Design review of the part built by this model. Coordinates are the model's own, in mm. Face numbers are marked on the shaded views. A direction names the side the tool comes from. Round coordinates to 2 decimals unless told otherwise and drop trailing zeros. Write each loop counter-clockwise with the first axis right and the second up, starting at its lowest first coordinate (ties: lowest second). Pieces come first, ordered by that corner, then holes.
from build123d import *

# Parameters (mm, degrees)
SCHIZZO1_R                   = 4
ESTRUSIONE_ESTRUSIONE1_DEPTH = 4
SCHIZZO2_R                   = 1.5
TAGLIO_ESTRUSIONE1_DEPTH     = 5
SCHIZZO3_R                   = 3.5
SCHIZZO3_R_2                 = 2
TAGLIO_ESTRUSIONE2_DEPTH     = 0.25
SCHIZZO4_R                   = 3
SCHIZZO4_R_2                 = 2
TAGLIO_ESTRUSIONE3_DEPTH     = 0.1
SCHIZZO5_R                   = 4.75
SCHIZZO5_R_2                 = 4
ESTRUSIONE_ESTRUSIONE2_DEPTH = 1
SCHIZZO6_W                   = 0.2
SCHIZZO6_H                   = 0.8


with BuildPart() as part:
    # Schizzo1 → Estrusione-Estrusione1 (new body)
    with BuildSketch(Plane.XY):
        Circle(SCHIZZO1_R)
    extrude(amount=ESTRUSIONE_ESTRUSIONE1_DEPTH)

    # Schizzo2 → Taglio-Estrusione1 (cut, through all)
    with BuildSketch(Plane.XY.offset(4)):
        Circle(SCHIZZO2_R)
    extrude(amount=-TAGLIO_ESTRUSIONE1_DEPTH, mode=Mode.SUBTRACT)

    # Schizzo3 → Taglio-Estrusione2 (cut)
    with BuildSketch(Plane(origin=(0, 0, 0), x_dir=(-1, 0, 0), z_dir=(0, 0, -1))):
        Circle(SCHIZZO3_R)
        Circle(SCHIZZO3_R_2, mode=Mode.SUBTRACT)
    taglio_estrusione2 = extrude(amount=-TAGLIO_ESTRUSIONE2_DEPTH, mode=Mode.SUBTRACT)

    # Schizzo4 → Taglio-Estrusione3 (cut)
    with BuildSketch(Plane(origin=(0, 0, 0.25), x_dir=(-1, 0, 0), z_dir=(0, 0, -1))):
        Circle(SCHIZZO4_R)
        Circle(SCHIZZO4_R_2, mode=Mode.SUBTRACT)
    taglio_estrusione3 = extrude(amount=-TAGLIO_ESTRUSIONE3_DEPTH, mode=Mode.SUBTRACT)

    # Specchia1: Taglio-Estrusione2, Taglio-Estrusione3 across plane
    add(taglio_estrusione2.mirror(Plane.XY.offset(2)), mode=Mode.SUBTRACT)
    add(taglio_estrusione3.mirror(Plane.XY.offset(2)), mode=Mode.SUBTRACT)

    # Schizzo5 → Estrusione-Estrusione2 (add)
    with BuildSketch(Plane.XY):
        Circle(SCHIZZO5_R)
        Circle(SCHIZZO5_R_2, mode=Mode.SUBTRACT)
    extrude(amount=ESTRUSIONE_ESTRUSIONE2_DEPTH)

    # Schizzo6 → Taglia-Rivoluzione1 (revolve, cut)
    with BuildSketch(Plane(origin=(0, 0, 0), x_dir=(1, 0, 0), z_dir=(0, 1, 0))):
        with Locations((3.9, -1.4)):
            Rectangle(SCHIZZO6_W, SCHIZZO6_H)
    revolve(axis=Axis((0, 0, 4), (0, 0, -1)), mode=Mode.SUBTRACT)


solid = part.part
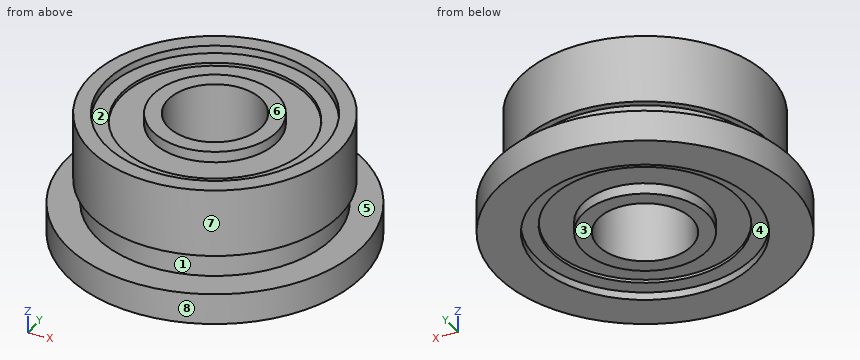
1) The part is to be moulded in two halves that separate along Y. For the marked faces 1, 2 and 3, say which applies: pulls with the +Y half, pulls with the -Y half, needs draft (parallel to the pull), parting line crosses it, or undercut.
2) For the marked faces 4, 5, 6, 7 and 8, list the 3-axis set-ups (+Z, -Z, +X, -X, +Y, -Y) from which the entire face can be reached by the end or side of a thin tool; tool diameter is ignored.
3) Add section B-B on z = 0.6. State the section outline as (x, y) points.
4) Add section C-C on z = 1.4. State the section outline as (x, y) points.
5) For line 1 along Y through (x, z) = (0, 0.3); line 2 along Y through (x, z) = (0, 3.9); line 3 along Y through (x, z) = (0, 2.05), list the stretches that pass through material, from the lowest coordinate up.
6) Add section A-A on y = -2.75. State the section outline as (x, z) points.
7) For P1, Ø1.5, axis at x = -2, z = 2.5, coming from the -Y side, flat-tipped, find the tip position at first contact; note if it passes through.
Computed:
1. face 1: parting line crosses it
1. face 2: undercut
1. face 3: needs draft
2. face 4: -Z
2. face 5: none
2. face 6: +Z, +X, -X, +Y, -Y
2. face 7: +Z
2. face 8: +Z, -Z
3. outline: circle Ø9.5 at (0, 0); hole circle Ø3 at (0, 0)
4. outline: circle Ø7.6 at (0, 0); hole circle Ø3 at (0, 0)
5. line 1: y = -4.75 to -3, -2 to -1.5, 1.5 to 2, 3 to 4.75
5. line 2: y = -4 to -3.5, -2 to -1.5, 1.5 to 2, 3.5 to 4
5. line 3: y = -4 to -1.5, 1.5 to 4
6. outline: (-3.87, 0) - (-2.17, 0) - (-2.17, 0.25) - (-1.2, 0.25) - (-1.2, 0.35) - (1.2, 0.35) - (1.2, 0.25) - (2.17, 0.25) - (2.17, 0) - (3.87, 0) - (3.87, 1) - (2.62, 1) - (2.62, 1.8) - (2.9, 1.8) - (2.9, 4) - (2.17, 4) - (2.17, 3.75) - (1.2, 3.75) - (1.2, 3.65) - (-1.2, 3.65) - (-1.2, 3.75) - (-2.17, 3.75) - (-2.17, 4) - (-2.9, 4) - (-2.9, 1.8) - (-2.62, 1.8) - (-2.62, 1) - (-3.87, 1) - close
7. P1: stops at y = -3.8
